Check sheet for the modelled part. Datum: model origin and axes. Units: mm. Round coordinates to 2 decimals unless told otherwise and drop trailing zeros. Write each loop counter-clockwise with the first axis right and the second up, starting at its lowest first coordinate (ties: lowest second). Pieces come first, ordered by that corner, then holes. Notation, with made-up numbers: M -29,16 L -6,16 A18 cw -6,44 Z; hole C 22,84 d3. An arc over 180 degrees is marked long. Put each result on its own line as item: value.
```python
from build123d import *

# Parameters (mm, degrees)
F1_DEPTH = 3.25


with BuildPart() as f1:
    # F0 (on Front) → F1 (new body, symmetric)
    with BuildSketch(Plane.XZ):
        with BuildLine():
            Line((12, 6.5), (12, 0))
            Line((12, 0), (-12, 0))
            Line((-12, 0), (-12, 6.5))
            Line((-12, 6.5), (-15, 6.5))
            Line((-15, 6.5), (-15, 13))
            Line((-15, 13), (-20, 13))
            ThreePointArc((-20, 13), (-26.655206, 3.42366), (-29, -8))
            Line((-29, -8), (-29, -65))
            Line((-29, -65), (-21, -65))
            Line((-21, -65), (-21, -20))
            ThreePointArc((-21, -20), (-17.485281, -11.514719), (-9, -8))
            Line((-9, -8), (9, -8))
            ThreePointArc((9, -8), (17.485281, -11.514719), (21, -20))
            Line((21, -20), (21, -65))
            Line((21, -65), (29, -65))
            Line((29, -65), (29, -8))
            ThreePointArc((29, -8), (26.655206, 3.42366), (20, 13))
            Line((20, 13), (15, 13))
            Line((15, 13), (15, 6.5))
            Line((15, 6.5), (12, 6.5))
        make_face()
    extrude(amount=F1_DEPTH, both=True)


solid = f1.part
```
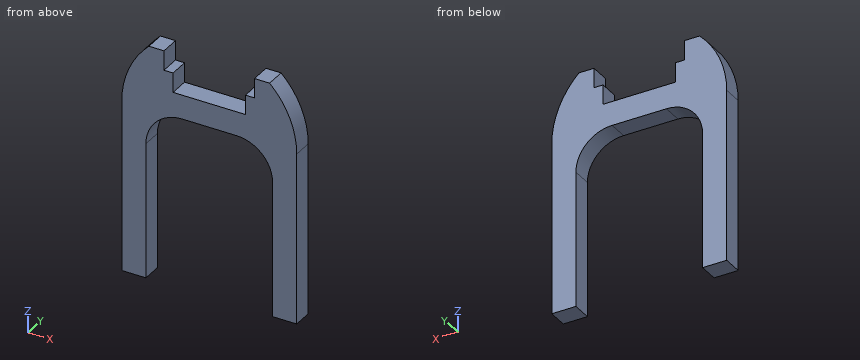
1. Cross-section at B-B (y = 0.75). Enter the section's corners in (x, z).
Computed values:
outline: M -29,-65 L -21,-65 L -21,-20 A12 cw -9,-8 L 9,-8 A12 cw 21,-20 L 21,-65 L 29,-65 L 29,-8 A29 ccw 20,13 L 15,13 L 15,6.5 L 12,6.5 L 12,0 L -12,0 L -12,6.5 L -15,6.5 L -15,13 L -20,13 A29 ccw -29,-8 Z
2. Scan lines: probe 1 along X at (y, z) = (-2, -42); probe 2 along X at (y, z) = (1, 0.5); probe 3 along Z at (x, y) = (-8, 0.75). Record each from-to range of solid material in increasing order.
Computed values:
probe 1: x = -29 to -21, 21 to 29
probe 2: x = -27.73 to -12, 12 to 27.73
probe 3: z = -8 to 0
3. Cross-section at C-C (z = -10.5). Enter the section's corners in (x, y).
Computed values:
outline: M -29,-3.25 L -16.33,-3.25 L -16.33,3.25 L -29,3.25 Z; M 16.33,-3.25 L 29,-3.25 L 29,3.25 L 16.33,3.25 Z
4. Cross-section at A-A (z = -32). Enter the section's corners in (x, y).
Computed values:
outline: M -29,-3.25 L -21,-3.25 L -21,3.25 L -29,3.25 Z; M 21,-3.25 L 29,-3.25 L 29,3.25 L 21,3.25 Z
5. Cross-section at D-D (x = -23.5). Enter the section's corners in (y, z), then the cut area to 3 significant figures.
Computed values:
outline: M -3.25,-65 L 3.25,-65 L 3.25,8.99 L -3.25,8.99 Z
area: 481 mm2
6. Depth check by flat-ended pin: pin 1 Ø3 at (x, y) = (-2, -1) entering from +Z; pin 2 Ø3 at (x, y) = (3.5, -1) entering from -Z; pin 3 Ø3 at (y, z) = (1.5, 10) entering from +X; pin 4 Ø1 at (x, z) = (-6.5, -9) entering from +Y. Enter the tip coordinate at first touch or a pass-through.
Computed values:
pin 1: stops at z = 0
pin 2: stops at z = -8
pin 3: stops at x = 23.85
pin 4: passes through
